Source: three-view drawing plus pictorial views. Frame: mm from the lowest corner of the part. A direction names the side the tool comes from. Round coordinates to 2 decimals unless told otherwise and drop trailing zeros. Loops run counter-clockwise (first coordinate to the right, second up) from the corner with the lowest first, then second, coordinate; pieces in that order, holes last. Notation, with made-up numbers: M 2,21.25 L 42,21.25 A23 cw 42,58.25 Z; hole C 52.5,66.25 d8. An arc over 180 degrees is marked long. Return JSON: item names as keys, results as strings. Group by question number.
1) Material intervals for line 1 (X direction, y = 0.25, z = 2.75); line 2 (X direction, y = 1.05, z = 0.5); line 3 (Z direction, x = 5.5, y = 1.35), sorted ascending. Write a range as from..to.
2) Section D-D (x = 3.25). Output: boundary loops of the cut face in (y, z), plus the area to 3 significant figures.
3) Contact query for flat-ended pins moving along their axis: P1, Ø0.9, axis at x = 3, y = 1.5, coming from the +Z side; P2, Ø0.9, axis at y = 1, z = 1.5, coming from the +X side. Output: stop coordinate, or through.
4) Section B-B (z = 7.2). Output: boundary loops of the cut face in (x, y), plus the area to 3 significant figures.
5) Access query for the marked faces 5, 6, 7, 8 and 9. Directions: +Z, -Z, +X, -X, +Y, -Y. A direction counts if a zero-diameter tool reaches every point of the face in a straight line with its end or side. Return the directions, or none.
6) Mould query, pull axis Z, two halves, no side actions, for the marked faces 1, 2, 3 and 4. Classes: +Z half, -Z half, draft (parallel to the pull), parting line (faces both ways), or undercut.
7) Section C-C (y = 1.05). Output: boundary loops of the cut face in (x, z).
8) Section A-A (x = 5.5). Output: boundary loops of the cut face in (y, z), plus the area to 3 significant figures.
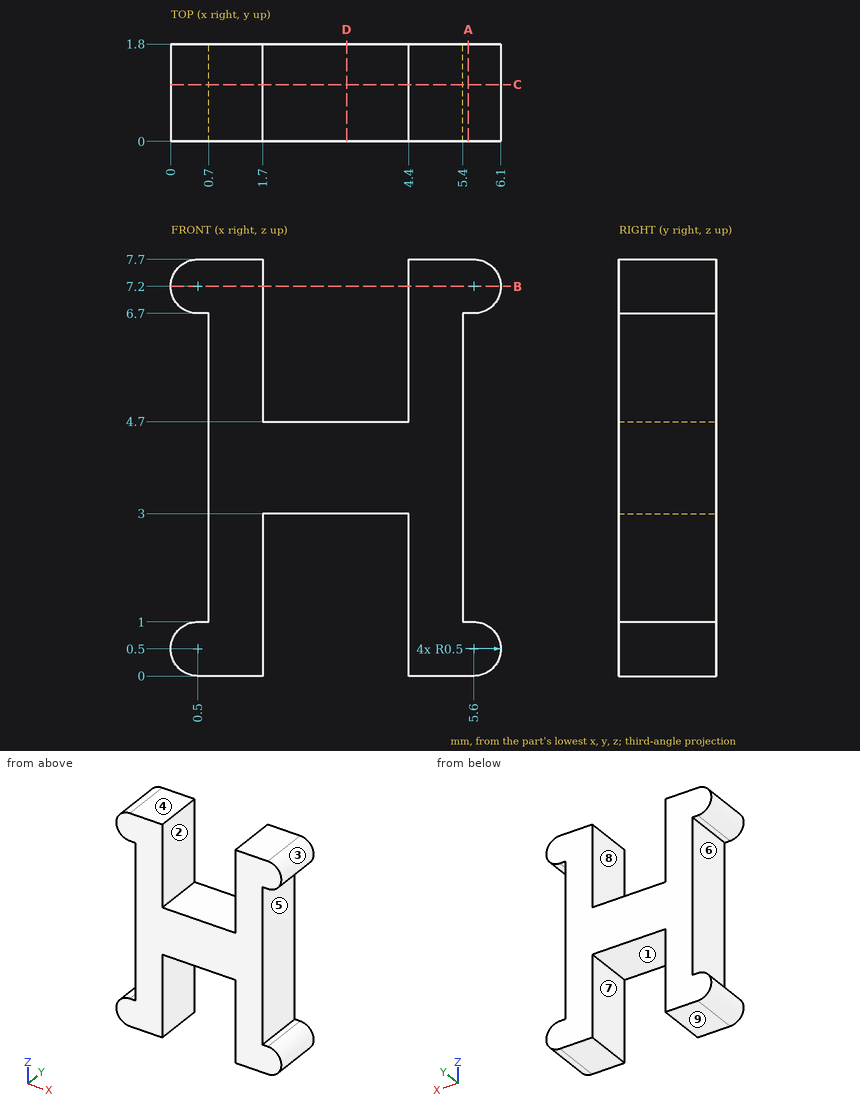
Returned:
{
 "1": {"line 1": "x = 0.7..1.7, 4.4..5.4", "line 2": "x = 0..1.7, 4.4..6.1", "line 3": "z = 0..1, 6.7..7.7"},
 "2": {"outline": "M 0,3 L 1.8,3 L 1.8,4.7 L 0,4.7 Z", "area": "3.06 mm^2"},
 "3": {"P1": "stops at z = 4.7", "P2": "stops at x = 5.4"},
 "4": {"outline": "M 0,0 L 1.7,0 L 1.7,1.8 L 0,1.8 Z; M 4.4,0 L 6.1,0 L 6.1,1.8 L 4.4,1.8 Z", "area": "6.12 mm^2"},
 "5": {"face 5": "+X, +Y, -Y", "face 6": "-X, +Y, -Y", "face 7": "-Z, +Y, -Y", "face 8": "+Z, +Y, -Y", "face 9": "-Z, +X, -X, +Y, -Y"},
 "6": {"face 1": "-Z half", "face 2": "draft", "face 3": "undercut", "face 4": "+Z half"},
 "7": {"outline": "M 0.5,0 L 1.7,0 L 1.7,3 L 4.4,3 L 4.4,0 L 5.6,0 A0.5 ccw 5.6,1 L 5.4,1 L 5.4,6.7 L 5.6,6.7 A0.5 ccw 5.6,7.7 L 4.4,7.7 L 4.4,4.7 L 1.7,4.7 L 1.7,7.7 L 0.5,7.7 A0.5 ccw 0.5,6.7 L 0.7,6.7 L 0.7,1 L 0.5,1 A0.5 ccw Z"},
 "8": {"outline": "M 0,0 L 1.8,0 L 1.8,1 L 0,1 Z; M 0,6.7 L 1.8,6.7 L 1.8,7.7 L 0,7.7 Z", "area": "3.60 mm^2"}
}
